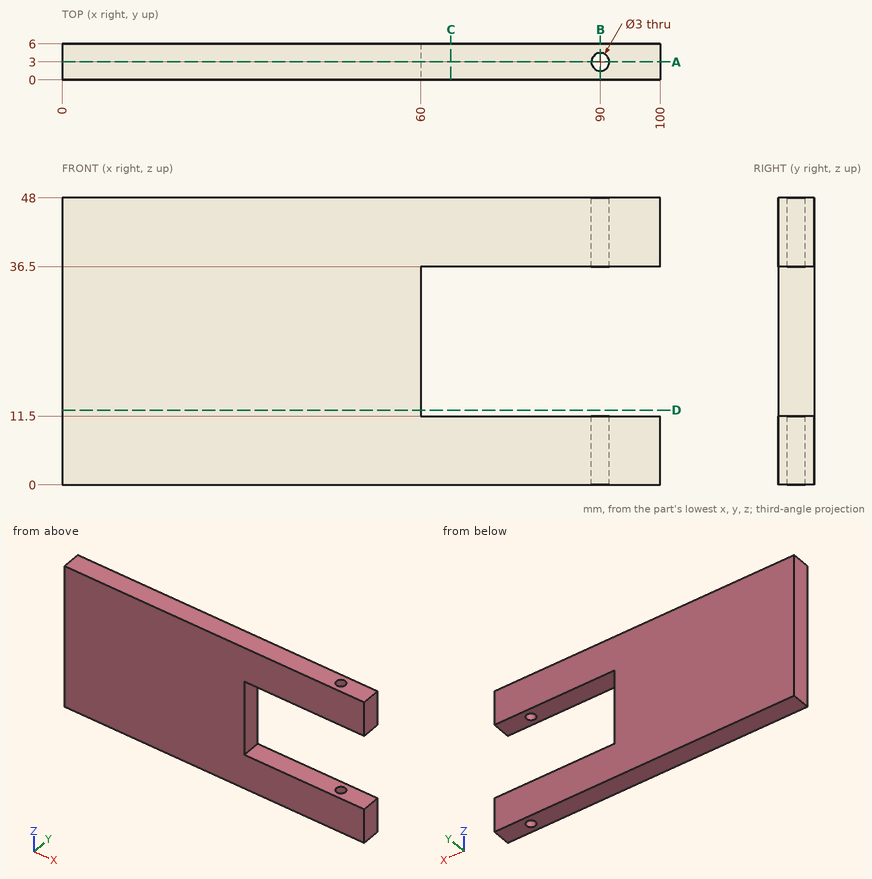
The drawing under review shows one solid part. Ordinate dimensions are in mm from its lowest x, y, z. Give positions to 0.01 mm unless a question says otherwise; leave off trailing zeros. Write each loop counter-clockwise with the first axis right and the second up, starting at its lowest first coordinate (ties: lowest second). Pieces come first, ordered by that corner, then holes. Notation, with made-up numbers: (47.25, -1) -> (51.25, -1) arc R23 cw to (51.25, 12) -> close; hole circle Ø10 at (-9, 22). An arc over 180 degrees is marked (long way). Answer in a Markdown table with one row per item.
(1) Clearance check with a flat-ended pin moving along its axis: pin 1 (3 mm diameter, centred on y = 2, z = 23, fed in from +X). State where the tip first meets the part, or that it passes through.
Results:
| item | result |
|---|---|
| pin 1 | x = 60 |
(2) Consider section C-C (x = 65). State the section outline as (y, z) points.
Results:
| item | result |
|---|---|
| outline | (0, 0) -> (6, 0) -> (6, 11.5) -> (0, 11.5) -> close; (0, 36.5) -> (6, 36.5) -> (6, 48) -> (0, 48) -> close |
(3) Consider section D-D (z = 12.5). State the section outline as (x, y) points, then the cut area to 3 significant figures.
Results:
| item | result |
|---|---|
| outline | (0, 0) -> (60, 0) -> (60, 6) -> (0, 6) -> close |
| area | 360 mm2 |
(4) Consider section B-B (x = 90). State the section outline as (y, z) points, then the cut area to 3 significant figures.
Results:
| item | result |
|---|---|
| outline | (0, 0) -> (1.5, 0) -> (1.5, 11.5) -> (0, 11.5) -> close; (0, 36.5) -> (1.5, 36.5) -> (1.5, 48) -> (0, 48) -> close; (4.5, 0) -> (6, 0) -> (6, 11.5) -> (4.5, 11.5) -> close; (4.5, 36.5) -> (6, 36.5) -> (6, 48) -> (4.5, 48) -> close |
| area | 69.0 mm2 |
(5) Consider section A-A (y = 3). State the section outline as (x, z) points.
Results:
| item | result |
|---|---|
| outline | (0, 0) -> (88.5, 0) -> (88.5, 11.5) -> (60, 11.5) -> (60, 36.5) -> (88.5, 36.5) -> (88.5, 48) -> (0, 48) -> close; (91.5, 0) -> (100, 0) -> (100, 11.5) -> (91.5, 11.5) -> close; (91.5, 36.5) -> (100, 36.5) -> (100, 48) -> (91.5, 48) -> close |
(6) To check wall thickness, follow probe 1 along Y at (x, z) = (90, 41.75); probe 2 along Z at (x, y) = (94, 2.45); probe 3 along X at (y, z) = (3, 44.75). State the ranges of each line that lie inside material, in increasing order.
Results:
| item | result |
|---|---|
| probe 1 | 0 to 1.5, 4.5 to 6 |
| probe 2 | 0 to 11.5, 36.5 to 48 |
| probe 3 | 0 to 88.5, 91.5 to 100 |
